```python
from build123d import *

# Parameters (mm, degrees)
ESQUISSE1_R                  = 1.047730405
ESQUISSE1_R_2                = 3.25
BOSS_EXTRU_1_DEPTH           = 3
BOSS_EXTRU_2_DEPTH           = 3
BOSS_EXTRU_2_DEPTH_BACK      = 3
ESQUISSE1_3_R                = 3.25
BOSS_EXTRU_3_DEPTH           = 6
BOSS_EXTRU_3_DEPTH_BACK      = 3
ESQUISSE1_4_R                = 3.25
BOSS_EXTRU_4_DEPTH           = 9
BOSS_EXTRU_4_DEPTH_BACK      = 3
ESQUISSE1_5_W                = 5.819303972
ESQUISSE1_5_H                = 10.5
ESQUISSE1_5_R                = 1.722458175
ESQUISSE1_5_R_2              = 1.751165812
ESQUISSE1_5_W_2              = 1.680696028
BOSS_EXTRU_5_DEPTH           = 8
BOSS_EXTRU_5_DEPTH_BACK      = 3
ESQUISSE1_6_R                = 1.751165812
ESQUISSE1_6_R_2              = 1.722458175
ENL_V_MAT_EXTRU_1_DEPTH      = 8
ENL_V_MAT_EXTRU_1_DEPTH_BACK = 8
CONG_1_R                     = 0.5


with BuildPart() as part:
    # Esquisse1 → Boss.-Extru.1 (new body)
    with BuildSketch(Plane.XY):
        Polygon((-21.5, -5.25), (-21.5, -6), (21.5, -6), (21.5, 6), (-21.5, 6), (-21.5, 5.25), (-15.680696028, 5.25), (-15.680696028, -5.25), align=None)
        with Locations((18.767939295, -2.963429097)):
            Circle(ESQUISSE1_R, mode=Mode.SUBTRACT)
        with Locations((-11.706099573, 2.280487387)):
            Circle(ESQUISSE1_R_2, mode=Mode.SUBTRACT)
        with Locations((12.713644898, 0)):
            Circle(ESQUISSE1_R_2, mode=Mode.SUBTRACT)
        with Locations((18.767939295, 3.012819582)):
            Circle(ESQUISSE1_R, mode=Mode.SUBTRACT)
    extrude(amount=-BOSS_EXTRU_1_DEPTH)

    # Esquisse1_3 → Boss.-Extru.2 (add, two sides: drawn at the far end of the back side and taken through both)
    with BuildSketch(Plane.XY.offset(-BOSS_EXTRU_2_DEPTH_BACK)):
        with Locations((-11.706099573, 2.280487387)):
            Circle(ESQUISSE1_3_R)
    extrude(amount=BOSS_EXTRU_2_DEPTH + BOSS_EXTRU_2_DEPTH_BACK)

    # Esquisse1_4 → Boss.-Extru.3 (add, two sides: drawn at the far end of the back side and taken through both)
    with BuildSketch(Plane.XY.offset(-BOSS_EXTRU_3_DEPTH_BACK)):
        with Locations((12.713644898, 0)):
            Circle(ESQUISSE1_4_R)
    extrude(amount=BOSS_EXTRU_3_DEPTH + BOSS_EXTRU_3_DEPTH_BACK)

    # Esquisse1_5 → Boss.-Extru.4 (add, two sides: drawn at the far end of the back side and taken through both)
    # profile 1 of 2: a face of its own
    with BuildSketch(Plane.XY.offset(-BOSS_EXTRU_4_DEPTH_BACK)):
        with Locations((-18.590348014, 0)):
            Rectangle(ESQUISSE1_5_W, ESQUISSE1_5_H)
        with Locations((-19.430696028, -2.963429097)):
            Circle(ESQUISSE1_5_R, mode=Mode.SUBTRACT)
        with Locations((-19.430696028, 3.012819582)):
            Circle(ESQUISSE1_5_R_2, mode=Mode.SUBTRACT)
    # profile 2 of 2: a face of its own
    with BuildSketch(Plane.XY.offset(-BOSS_EXTRU_4_DEPTH_BACK)):
        with Locations((-22.340348014, 0)):
            Rectangle(ESQUISSE1_5_W_2, ESQUISSE1_5_H)
    extrude(amount=BOSS_EXTRU_4_DEPTH + BOSS_EXTRU_4_DEPTH_BACK)

    # Esquisse1_6 → Boss.-Extru.5 (add, two sides: drawn at the far end of the back side and taken through both)
    with BuildSketch(Plane.XY.offset(-BOSS_EXTRU_5_DEPTH_BACK)):
        with Locations((-19.430696028, 3.012819582)):
            Circle(ESQUISSE1_6_R)
        with Locations((-19.430696028, -2.963429097)):
            Circle(ESQUISSE1_6_R_2)
    extrude(amount=BOSS_EXTRU_5_DEPTH + BOSS_EXTRU_5_DEPTH_BACK)

    # Esquisse2 → Enl_v. mat.-Extru.1 (cut, two sides: drawn at the far end of the back side and taken through both)
    with BuildSketch(Plane(origin=(0, 0, 0), x_dir=(1, 0, 0), z_dir=(0, 1, 0)).offset(-ENL_V_MAT_EXTRU_1_DEPTH_BACK)):
        Polygon((-23.180696028, -5.790746035), (-22.293736237, -9), (-23.180696028, -9), align=None)
        Polygon((-15.680696028, -6.586297382), (-16.769074106, -9), (-15.680696028, -9), align=None)
    extrude(amount=ENL_V_MAT_EXTRU_1_DEPTH + ENL_V_MAT_EXTRU_1_DEPTH_BACK, mode=Mode.SUBTRACT)

    # Cong_1
    cong_1_edges = [part.edges().sort_by_distance(p)[0] for p in [
        (9.463644898, 0, 6),
    ]]
    fillet(cong_1_edges, radius=CONG_1_R)


solid = part.part
```
Build history of the part. All positions in model axes, mm. A direction names the side the tool comes from. Round coordinates to 2 decimals unless told otherwise and drop trailing zeros. Write each loop counter-clockwise with the first axis right and the second up, starting at its lowest first coordinate (ties: lowest second). Pieces come first, ordered by that corner, then holes. Notation, with made-up numbers: (79, 0.25) - (85, 0.25) arc R30 ccw to (85, 34.25) - close; hole circle Ø3 at (80.5, 14.25). An arc over 180 degrees is marked (long way). Answer as CSV lines item,"result".
Q1. Drill centre lines: probe 1 along X at (y, z) = (0.75, 1.5); probe 2 along Z at (x, y) = (-15.5, 2.25); probe 3 along X at (y, z) = (-2.75, 4.5). Where is each one in solid material? Low to high. Write a range as [from, to].
Report:
probe 1,"x = [-23.18, -15.68], [-14.57, -8.84], [9.55, 15.88]"
probe 2,"z = [-3, 0]"
probe 3,"x = [-23.18, -15.68], [10.98, 14.45]"
Q2. Cut at C-C (z = 1.25). Write the cut outline in (x, y).
Report:
outline,"(-23.18, -5.25) - (-15.68, -5.25) - (-15.68, 5.25) - (-23.18, 5.25) - close; circle Ø6.5 at (-11.71, 2.28); circle Ø6.5 at (12.71, 0)"
Q3. Cut at D-D (x = 5.5). Write the cut outline in (y, z).
Report:
outline,"(-6, -3) - (6, -3) - (6, 0) - (-6, 0) - close"
Q4. Tool access for faces 1 (the flat face through (-12, 2, 3)), 2 (the cylindrical face through (18.5, 2, -1.5)), 3 (the cylindrical face through (15.716, -1.245, 2.712)), 4 (the flat face through (13, 0, 6)): list every direction of +Z, -Z, +X, -X, +Y, -Y with a clear straight run to the whole face (end or side of a thin tool).
Report:
face 1,"+Z, +Y, -Y"
face 2,"+Z, -Z"
face 3,"+Z"
face 4,"+Z, +X, +Y, -Y"
Q5. Drop flat-ended pins along their axis: pin 1 (5 mm diameter, centred on x = -13, y = 1.5, fed in from +Z); pin 2 (6 mm diameter, centred on x = -21, z = 5.5, fed in from -Y); pin 3 (2 mm diameter, centred on y = 0, z = 4, fed in from +X). Give the stop position or say it passes through.
Report:
pin 1,"stops at z = 3"
pin 2,"stops at y = -5.25"
pin 3,"stops at x = 15.96"
Q6. Cut at A-A (z = 3.75). Write the cut outline in (x, y).
Report:
outline,"(-23.18, -5.25) - (-15.68, -5.25) - (-15.68, 5.25) - (-23.18, 5.25) - close; circle Ø6.5 at (12.71, 0)"
Q7. Cut at B-B (y = 0). Write the cut outline in (x, z), and give its area (3 significant figures).
Report:
outline,"(-23.18, -3) - (21.5, -3) - (21.5, 0) - (15.96, 0) - (15.96, 5.5) arc R0.5 ccw to (15.46, 6) - (9.96, 6) arc R0.5 ccw to (9.46, 5.5) - (9.46, 0) - (-9.39, 0) - (-9.39, 3) - (-14.02, 3) - (-14.02, 0) - (-15.68, 0) - (-15.68, 6.59) - (-16.77, 9) - (-22.29, 9) - (-23.18, 5.79) - close"
area,"252 mm^2"
Q8. Pull direction X, two halves, no side cores. Call faces 5 (the flat face through (0, -6, -1)), 6 (the flat face through (-16.22, -0.07, 7.78)), 7 (the flat face through (0, 0, 0)): +X half, -X half, draft (parallel to the pull), parting line (faces both ways), or undercut.
Report:
face 5,"draft"
face 6,"+X half"
face 7,"undercut"
